Here's how the part is built. I have some questions about the finished solid (model axes, mm). Face numbers are marked on the shaded views. A direction names the side the tool comes from. Coordinates: 2 decimals unless noted, no trailing zeros. Write each loop counter-clockwise with the first axis right and the second up, starting at its lowest first coordinate (ties: lowest second). Pieces come first, ordered by that corner, then holes.
Item 1: If we section it at C-C (x = 38.5): Please give me the cut outline in (y, z).
Item 2: If we section it at B-B (y = -1.75): Please give me the cut outline in (x, z) (3 decimals), then the cut area to 3 significant figures.
Item 3: If we section it at D-D (x = 16.1): Please give me the cut outline in (y, z) (1 decimal), then the cut area to 3 significant figures.
Item 4: If I drill on line 1 (X direction, y = -3, z = -10) (3 decimals); line 2 (Z direction, x = 71.3, y = -5) (3 decimals); line 3 (Z direction, x = 16.1, y = -5.75) (3 decimals), over which ranges is the centre line in solid material (lowest first)?
Item 5: For the marked faces 4 and 5, which set-ups out of +Z, -Z, +X, -X, +Y, -Y let a thin tool reach every point of the face, with its end or its side?
Item 6: If we section it at A-A (z = -10): Please give me the cut outline in (x, y) (3 decimals).
Item 7: I'm going to push flat-ended pins straight in: pin 1 Ø4 at (y, z) = (-17, 11.5) entering from -X; pin 2 Ø1.5 at (x, z) = (77.5, 3) entering from -Y; pin 3 Ø2 at (x, y) = (43, -2) entering from +Z (3 decimals); pin 4 Ø3 at (x, z) = (62.5, -9.5) entering from -Y. Where does each tip first touch, or does it pass through?
Item 8: We'd pull the mould along X, two halves only. Please class the marked faces 1, 2 and 3: +X half, -X half, draft (parallel to the pull), parting line (faces both ways), or undercut.
from build123d import *

# Parameters (mm, degrees)
BOSS_EXTRUDE1_DEPTH = 87
SKETCH2_R           = 3.175
CUT_EXTRUDE1_DEPTH  = 21
FILLET1_R           = 5


with BuildPart() as part:
    # Sketch1 → Boss-Extrude1 (new body)
    with BuildSketch(Plane(origin=(0, 0, 0), x_dir=(0, 0, -1), z_dir=(1, 0, 0))):
        with BuildLine():
            Line((-32.5, 0), (-25, 0))
            ThreePointArc((-25, 0), (-12.5, -12.5), (0, 0))
            Line((0, 0), (20, 0))
            Line((20, 0), (20, -10))
            Line((20, -10), (4.820508076, -10))
            ThreePointArc((4.820508076, -10), (-17.676380902, -19.318516526), (-32.5, 0))
        make_face()
    extrude(amount=BOSS_EXTRUDE1_DEPTH)

    # Sketch2 → Cut-Extrude1 (cut, through all)
    with BuildSketch(Plane(origin=(0, 0, 0), x_dir=(1, 0, 0), z_dir=(0, 1, 0))):
        with Locations((71.3, 10)):
            Circle(SKETCH2_R)
        with Locations((16.1, 10)):
            Circle(SKETCH2_R)
    extrude(amount=-CUT_EXTRUDE1_DEPTH, mode=Mode.SUBTRACT)

    # Fillet1
    fillet1_edges = [part.edges().sort_by_distance(p)[0] for p in [
        (43.5, -10, -20),
    ]]
    fillet(fillet1_edges, radius=FILLET1_R)


solid = part.part
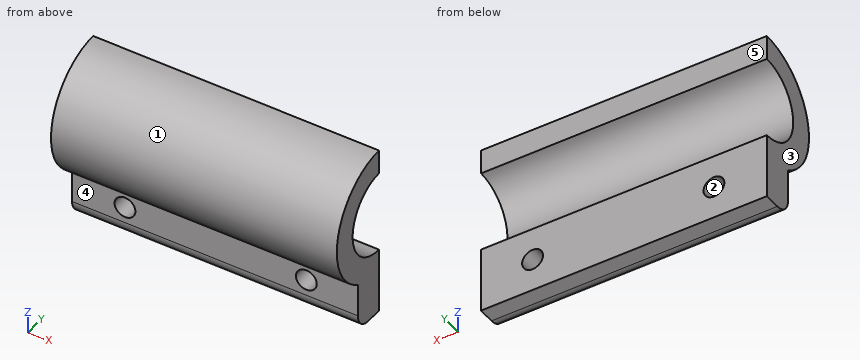
Answer list:
1. outline: (-10, -15) arc R5 ccw to (-5, -20) - (0, -20) - (0, 0) arc R12.5 cw to (0, 25) - (0, 32.5) arc R20 ccw to (-10, -4.82) - close
2. outline: (0, -20) - (87, -20) - (87, 0.123) - (0, 0.123) - close; (0, 24.877) - (87, 24.877) - (87, 32.423) - (0, 32.423) - close; hole circle Ø6.35 at (16.1, -10); hole circle Ø6.35 at (71.3, -10)
2. area: 2,340 mm2
3. outline: (-10, -15) arc R5 ccw to (-5, -20) - (0, -20) - (0, -13.2) - (-10, -13.2) - close; (-10, -6.8) - (0, -6.8) - (0, 0) arc R12.5 cw to (0, 25) - (0, 32.5) arc R20 ccw to (-10, -4.8) - close
3. area: 448 mm2
4. line 1: x = 0 to 12.925, 19.275 to 68.125, 74.475 to 87
4. line 2: z = -20 to -13.175, -6.825 to 1.044, 23.956 to 31.865
4. line 3: z = -19.943 to -13.175, -6.825 to 1.401, 23.599 to 31.656
5. face 4: -Z, +X, -X, -Y
5. face 5: +Z, -Z, +X, -X, +Y
6. outline: (0, -10) - (12.925, -10) - (12.925, 0) - (0, 0) - close; (19.275, -10) - (68.125, -10) - (68.125, 0) - (19.275, 0) - close; (74.475, -10) - (87, -10) - (87, 0) - (74.475, 0) - close
7. pin 1: stops at x = 0
7. pin 2: stops at y = -17.98
7. pin 3: stops at z = 32.475
7. pin 4: stops at y = -10
8. face 1: draft
8. face 2: undercut
8. face 3: -X half
